Could you check a few things on this model? Use its own coordinates, in mm. Face numbers are marked on the shaded views. A direction names the side the tool comes from. Give positions to 0.01 mm unless a question says otherwise; leave off trailing zeros. Order: outer loops, then holes, each group sorted by start corner. A loop starts at its lowest first (then second) coordinate and runs counter-clockwise, first axis right, second up. Notation, with made-up numbers: (85.5, 4) - (130.5, 4) arc R29 ccw to (130.5, 41) - close; hole circle Ø8 at (49.25, 57.25). An arc over 180 degrees is marked (long way). One line per question, with ' | ' between items. Start each with the question number.
1. I need wall thicknesses on probe 1 along X at (y, z) = (1.6, 0); probe 2 along X at (y, z) = (1.1, 15); probe 3 along Y at (x, z) = (16, -35). Which ranges of each line are inside material? Lowest first, please. Write a range as from..to.
2. For P1, Ø2, axis at y = 32, z = -35.5, coming from the -X side; P2, Ø6, axis at y = 10, z = -18.5, coming from the -X side; P3, Ø3.5, axis at x = -35, y = 6, coming from the +Z side, each with a flat end and sliding along its axis, tell me the tip position at first contact or that it passes through.
3. If we mould it in two halves opening along Z, with no side actions, what happens to the marked faces 1 and 2? For each: released by +Z, released by -Z, zero draft, split by the parting line, or undercut.
4. Which directions (+Z, -Z, +X, -X, +Y, -Y) give clear straight access to the entire face, cutting with the end or side of a thin tool? Please do the marked faces 3 and 4.
5. Imagine slicing it at B-B (z = 0). Please give me the cut outline in (x, y), and give its area (3 significant figures).
6. Imagine slicing it at A-A (x = 0). Please give me the cut outline in (y, z).
7. Imagine slicing it at C-C (y = 32). Please give me the cut outline in (x, z), and give its area (3 significant figures).
8. Imagine slicing it at D-D (x = 16). Please give me the cut outline in (y, z), and give its area (3 significant figures).
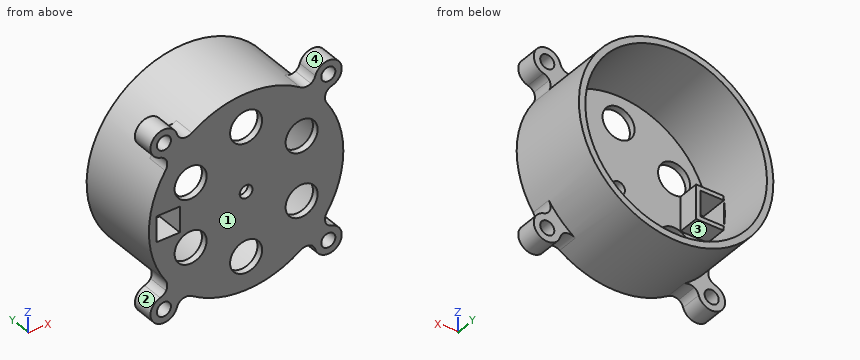
```python
from build123d import *

# Parameters (mm, degrees)
SKETCH1_R               = 45.5
BOSS_EXTRUDE1_DEPTH     = 40
SHELL1_T                = -3
CUT_EXTRUDE2_DEPTH      = 76.766087401
CUT_EXTRUDE2_DEPTH_BACK = 76.766087401
SKETCH3_R               = 7.5
SKETCH4_R               = 3
CUT_EXTRUDE3_DEPTH      = 3
SKETCH6_W               = 15
SKETCH6_H               = 16
SKETCH6_W_2             = 11
SKETCH6_H_2             = 12
BOSS_EXTRUDE2_DEPTH     = 10
SKETCH7_W               = 11
SKETCH7_H               = 12
CUT_EXTRUDE5_DEPTH      = 3
SKETCH8_R               = 3.3
BOSS_EXTRUDE3_DEPTH     = 10
CIRPATTERN1_COUNT       = 4
FILLET1_R               = 5


with BuildPart() as part:
    # Sketch1 → Boss-Extrude1 (new body)
    with BuildSketch(Plane(origin=(0, 0, 0), x_dir=(1, 0, 0), z_dir=(0, 1, 0))):
        with Locations(Location((0, 0, 0), (0, 0, 270))):
            Circle(SKETCH1_R)
    extrude(amount=BOSS_EXTRUDE1_DEPTH)

    # Shell1
    shell1_openings = [part.faces().sort_by_distance(p)[0] for p in [
        (0, 40, 0),
    ]]
    offset(amount=SHELL1_T, openings=shell1_openings, kind=Kind.INTERSECTION)

    # Sketch3 → Cut-Extrude2 (cut, two sides: drawn at the far end of the back side and taken through both)
    with BuildSketch(Plane.XZ.offset(-CUT_EXTRUDE2_DEPTH_BACK)):
        with Locations(Location((0, 30, 0), (0, 0, 90))):
            Circle(SKETCH3_R)
        with Locations(Location((25.980762114, 15, 0), (0, 0, 90))):
            Circle(SKETCH3_R)
        with Locations(Location((25.980762114, -15, 0), (0, 0, 90))):
            Circle(SKETCH3_R)
        with Locations(Location((0, -30, 0), (0, 0, 90))):
            Circle(SKETCH3_R)
        with Locations(Location((-25.980762114, -15, 0), (0, 0, 90))):
            Circle(SKETCH3_R)
        with Locations(Location((-25.980762114, 15, 0), (0, 0, 90))):
            Circle(SKETCH3_R)
    extrude(amount=CUT_EXTRUDE2_DEPTH + CUT_EXTRUDE2_DEPTH_BACK, mode=Mode.SUBTRACT)

    # Sketch4 → Cut-Extrude3 (cut)
    with BuildSketch(Plane(origin=(0, 3, 0), x_dir=(1, 0, 0), z_dir=(0, 1, 0))):
        with Locations(Location((0, 0, 0), (0, 0, 270))):
            Circle(SKETCH4_R)
    extrude(amount=-CUT_EXTRUDE3_DEPTH, mode=Mode.SUBTRACT)

    # Sketch6 → Boss-Extrude2 (add)
    with BuildSketch(Plane(origin=(0, 3, 0), x_dir=(1, 0, 0), z_dir=(0, 1, 0))):
        with Locations((-36.5, 0)):
            Rectangle(SKETCH6_W, SKETCH6_H)
        with Locations((-36.5, 0)):
            Rectangle(SKETCH6_W_2, SKETCH6_H_2, mode=Mode.SUBTRACT)
    extrude(amount=BOSS_EXTRUDE2_DEPTH)

    # Sketch7 → Cut-Extrude5 (cut)
    with BuildSketch(Plane(origin=(0, 3, 0), x_dir=(1, 0, 0), z_dir=(0, 1, 0))):
        with Locations((-36.5, 0)):
            Rectangle(SKETCH7_W, SKETCH7_H)
    extrude(amount=-CUT_EXTRUDE5_DEPTH, mode=Mode.SUBTRACT)

    # Sketch8 → Boss-Extrude3 (add)
    with BuildSketch(Plane(origin=(0, 0, 0), x_dir=(1, 0, 0), z_dir=(0, 1, 0))):
        with BuildLine():
            Line((32.166608897, 38.466608897), (27.854823504, 35.97719844))
            ThreePointArc((27.854823504, 35.97719844), (32.173358544, 32.173358544), (35.97719844, 27.854823504))
            Line((35.97719844, 27.854823504), (38.466608897, 32.166608897))
            ThreePointArc((38.466608897, 32.166608897), (42.921381618, 42.921381618), (32.166608897, 38.466608897))
        make_face()
        with Locations(Location((38.466608897, 38.466608897, 0), (0, 0, 270))):
            Circle(SKETCH8_R, mode=Mode.SUBTRACT)
    boss_extrude3 = extrude(amount=BOSS_EXTRUDE3_DEPTH)

    # CirPattern1: Boss-Extrude3 ×4 about axis
    cirpattern1_axis = Axis((0, 0, 0), (0, 1, 0))
    for i in range(1, CIRPATTERN1_COUNT):
        add(boss_extrude3.rotate(cirpattern1_axis, i * 360 / CIRPATTERN1_COUNT))

    # Fillet1
    # the kernel refuses this fillet: 5 mm, written as the material it adds along each edge
    with BuildSketch(Plane(origin=(-38.466608897, 0, 32.166608897), x_dir=(0.5000000000000063, 0, -0.866025403784435), z_dir=(0, 1, 0)), Plane(origin=(32.166608897, 0, 38.466608897), x_dir=(-0.8660254037844374, 0, -0.5000000000000022), z_dir=(0, 1, 0)), Plane(origin=(38.466608897, 0, -32.166608897), x_dir=(-0.5000000000000032, 0, 0.8660254037844368), z_dir=(0, 1, 0)), Plane(origin=(-32.166608897, 0, -38.466608897), x_dir=(0.8660254037844356, 0, 0.5000000000000054), z_dir=(0, 1, 0))) as fillet1_piece_1:
        with BuildLine():
            CenterArc((2.371395832, 5), FILLET1_R, 226.156864412, 43.843135588)
            ThreePointArc((-1.092035972, 1.39380531), (-0.496806454, 0.735459519), (0, 0))
            Line((0, 0), (2.371395832, 0))
        make_face()
    extrude(amount=10)
    with BuildSketch(Plane(origin=(-32.166608897, 0, 38.466608897), x_dir=(0.8660254037844327, 0, -0.5000000000000103), z_dir=(0, 1, 0)), Plane(origin=(38.466608897, 0, 32.166608897), x_dir=(-0.5000000000000117, 0, -0.8660254037844319), z_dir=(0, 1, 0)), Plane(origin=(32.166608897, 0, -38.466608897), x_dir=(-0.8660254037844319, 0, 0.5000000000000117), z_dir=(0, 1, 0)), Plane(origin=(-38.466608897, 0, -32.166608897), x_dir=(0.500000000000011, 0, 0.8660254037844324), z_dir=(0, 1, 0))) as fillet1_piece_2:
        with BuildLine():
            CenterArc((2.371395832, -5), FILLET1_R, 90, 43.843135588)
            ThreePointArc((-1.092035972, -1.39380531), (-0.496806454, -0.735459519), (0, 0))
            Line((0, 0), (2.371395832, 0))
        make_face()
    extrude(amount=10)
    with BuildSketch(Plane(origin=(-27.854823504, 0, 35.97719844), x_dir=(0.8108999282777639, 0, 0.5851848479917412), z_dir=(0, 1, 0)), Plane(origin=(35.97719844, 0, 27.854823504), x_dir=(0.5851848479917567, 0, -0.8108999282777527), z_dir=(0, 1, 0)), Plane(origin=(27.854823504, 0, -35.97719844), x_dir=(-0.8108999282777679, 0, -0.5851848479917359), z_dir=(0, 1, 0)), Plane(origin=(-35.97719844, 0, -27.854823504), x_dir=(-0.5851848479917252, 0, 0.8108999282777755), z_dir=(0, 1, 0))) as fillet1_piece_3:
        with BuildLine():
            CenterArc((3.236915302, -4.997156955), FILLET1_R, 91.932257762, 63.883791986)
            Line((-1.32425924, -2.948819386), (0, 0))
            ThreePointArc((0, 0), (1.534162982, -0.025871708), (3.068325963, 0))
        make_face()
    extrude(amount=10)
    with BuildSketch(Plane(origin=(-35.97719844, 0, 27.854823504), x_dir=(-0.5851848479917389, 0, -0.8108999282777657), z_dir=(0, 1, 0)), Plane(origin=(27.854823504, 0, 35.97719844), x_dir=(-0.8108999282777541, 0, 0.5851848479917549), z_dir=(0, 1, 0)), Plane(origin=(35.97719844, 0, -27.854823504), x_dir=(0.5851848479917436, 0, 0.8108999282777621), z_dir=(0, 1, 0)), Plane(origin=(-27.854823504, 0, -35.97719844), x_dir=(0.8108999282777745, 0, -0.5851848479917268), z_dir=(0, 1, 0))) as fillet1_piece_4:
        with BuildLine():
            CenterArc((3.236915302, 4.997156955), FILLET1_R, 204.183950253, 63.883791986)
            Line((-1.32425924, 2.948819386), (0, 0))
            ThreePointArc((0, 0), (1.534162982, 0.025871708), (3.068325963, 0))
        make_face()
    extrude(amount=10)


solid = part.part
```
Results found:
1) probe 1: x = -45.5..-42, -31..-3, 3..45.5 | probe 2: x = -42.96..-33.48, -18.48..18.48, 33.48..42.96 | probe 3: y = 0..3
2) P1: stops at x = -29.66 | P2: stops at x = -42.78 | P3: stops at z = 44.53
3) face 1: zero draft | face 2: undercut
4) face 3: +Y | face 4: +Y, -Y
5) outline: (-45.5, 0) - (-42, 0) - (-42, 13) - (-42.5, 13) - (-42.5, 40) - (-45.5, 40) - close; (-31, 0) - (-3, 0) - (-3, 3) - (-29, 3) - (-29, 13) - (-31, 13) - close; (3, 0) - (45.5, 0) - (45.5, 40) - (42.5, 40) - (42.5, 3) - (3, 3) - close | area: 469 mm2
6) outline: (0, -45.5) - (40, -45.5) - (40, -42.5) - (3, -42.5) - (3, -37.5) - (0, -37.5) - close; (0, -22.5) - (3, -22.5) - (3, -3) - (0, -3) - close; (0, 3) - (3, 3) - (3, 22.5) - (0, 22.5) - close; (0, 37.5) - (3, 37.5) - (3, 42.5) - (40, 42.5) - (40, 45.5) - (0, 45.5) - close
7) outline: circle Ø91 at (0, 0); hole circle Ø85 at (0, 0) | area: 829 mm2
8) outline: (0, -42.59) - (40, -42.59) - (40, -39.37) - (3, -39.37) - (3, 39.37) - (40, 39.37) - (40, 42.59) - (0, 42.59) - close | area: 494 mm2
